from build123d import *

# Parameters (mm, degrees)
SKETCH3_R            = 2.75
BOSS_EXTRUDE1_DEPTH  = 3
SKETCH4_R            = 2.75
BOSS_EXTRUDE2_DEPTH  = 3
BOSS_EXTRUDE3_DEPTH  = 3
BOSS_EXTRUDE4_START  = -3
SKETCH6_R            = 2.75
BOSS_EXTRUDE4_DEPTH  = 3
CUT_EXTRUDE1_START   = -0.4
CUT_EXTRUDE1_DEPTH   = 0.4
CUT_EXTRUDE2_DEPTH   = 0.4
BOSS_EXTRUDE5_DEPTH  = 26
SKETCH11_W           = 1.5
SKETCH11_H           = 10.4
CUT_EXTRUDE4_DEPTH   = 9.5
SKETCH13_W           = 13.75
SKETCH13_H           = 0.5
BOSS_EXTRUDE6_DEPTH  = 1
BOSS_EXTRUDE7_DEPTH  = 1
BOSS_EXTRUDE8_DEPTH  = 3
CHAMFER1_SIZE        = 2
FILLET1_R            = 1
SKETCH16_W           = 26
SKETCH16_H           = 3
BOSS_EXTRUDE9_DEPTH  = 1
FILLET2_R            = 2
BOSS_EXTRUDE11_DEPTH = 2.4
BOSS_EXTRUDE12_DEPTH = 1
CUT_EXTRUDE5_DEPTH   = 0.5


with BuildPart() as part:
    # Sketch3 → Boss-Extrude1 (new body)
    with BuildSketch(Plane(origin=(10, 0, 0), x_dir=(0, 0, -1), z_dir=(1, 0, 0))):
        with BuildLine():
            Line((-37, 41.45), (-42, 41.45))
            Line((-42, 41.45), (-47, 41.45))
            Line((-47, 41.45), (-47, 34.45))
            ThreePointArc((-47, 34.45), (-46.121320344, 32.328679656), (-44, 31.45))
            Line((-44, 31.45), (-40, 31.45))
            ThreePointArc((-40, 31.45), (-37.878679656, 32.328679656), (-37, 34.45))
            Line((-37, 34.45), (-37, 41.45))
        make_face()
        with Locations((-42, 36.65)):
            Circle(SKETCH3_R, mode=Mode.SUBTRACT)
    extrude(amount=BOSS_EXTRUDE1_DEPTH)

    # Sketch6 → Boss-Extrude4 (add)
    with BuildSketch(Plane(origin=(13, 0, 0), x_dir=(0, 0, -1), z_dir=(1, 0, 0)).offset(BOSS_EXTRUDE4_START)):
        with BuildLine():
            Line((-36.6, 31.45), (-36.6, 41.45))
            Line((-36.6, 41.45), (-47, 41.45))
            Line((-47, 41.45), (-47, 34.45))
            ThreePointArc((-47, 34.45), (-46.121320344, 32.328679656), (-44, 31.45))
            Line((-44, 31.45), (-36.6, 31.45))
        make_face()
        with Locations(Location((-42, 36.65, 0), (0, 0, 180))):
            Circle(SKETCH6_R, mode=Mode.SUBTRACT)
    extrude(amount=BOSS_EXTRUDE4_DEPTH)

    # Sketch8 → Cut-Extrude2 (cut)
    with BuildSketch(Plane.ZY.offset(-10)):
        with BuildLine():
            Line((47, 41.45), (36.6, 41.45))
            Line((36.6, 41.45), (36.6, 31.45))
            Line((36.6, 31.45), (44, 31.45))
            ThreePointArc((44, 31.45), (46.121320344, 32.328679656), (47, 34.45))
            Line((47, 34.45), (47, 41.45))
        make_face()
    extrude(amount=-CUT_EXTRUDE2_DEPTH, mode=Mode.SUBTRACT)



with BuildPart() as body_2:
    # Sketch4 → Boss-Extrude2 (new body)
    with BuildSketch(Plane.ZY.offset(10)):
        with BuildLine():
            Line((47, 41.45), (37, 41.45))
            Line((37, 41.45), (37, 34.45))
            ThreePointArc((37, 34.45), (37.878679656, 32.328679656), (40, 31.45))
            Line((40, 31.45), (44, 31.45))
            ThreePointArc((44, 31.45), (46.121320344, 32.328679656), (47, 34.45))
            Line((47, 34.45), (47, 41.45))
        make_face()
        with Locations((42, 36.65)):
            Circle(SKETCH4_R, mode=Mode.SUBTRACT)
    extrude(amount=BOSS_EXTRUDE2_DEPTH)

    # Sketch5 → Boss-Extrude3 (add)
    with BuildSketch(Plane.ZY.offset(13)):
        with BuildLine():
            Line((37, 41.45), (36.6, 41.45))
            Line((36.6, 41.45), (36.6, 31.45))
            Line((36.6, 31.45), (40, 31.45))
            ThreePointArc((40, 31.45), (37.878679656, 32.328679656), (37, 34.45))
            Line((37, 34.45), (37, 41.45))
        make_face()
    extrude(amount=-BOSS_EXTRUDE3_DEPTH)

    # Sketch7 → Cut-Extrude1 (cut)
    with BuildSketch(Plane(origin=(-10, 0, 0), x_dir=(0, 0, -1), z_dir=(1, 0, 0)).offset(CUT_EXTRUDE1_START)):
        with BuildLine():
            Line((-36.6, 41.45), (-47, 41.45))
            Line((-47, 41.45), (-47, 34.45))
            ThreePointArc((-47, 34.45), (-46.121320344, 32.328679656), (-44, 31.45))
            Line((-44, 31.45), (-36.6, 31.45))
            Line((-36.6, 31.45), (-36.6, 41.45))
        make_face()
    extrude(amount=CUT_EXTRUDE1_DEPTH, mode=Mode.SUBTRACT)


with BuildPart() as part_1:
    add(part.part)

    add(body_2.part)  # Boss-Extrude5 merges body 2
    # Sketch9 → Boss-Extrude5 (add)
    with BuildSketch(Plane(origin=(13, 0, 0), x_dir=(0, 0, -1), z_dir=(1, 0, 0))):
        with BuildLine():
            ThreePointArc((-31.6, 41.45), (-35.135533906, 39.985533906), (-36.6, 36.45))
            Line((-36.6, 36.45), (-34.35, 36.45))
            ThreePointArc((-34.35, 36.45), (-31.6, 39.2), (-28.85, 36.45))
            Line((-28.85, 36.45), (-26.6, 36.45))
            ThreePointArc((-26.6, 36.45), (-28.064466094, 39.985533906), (-31.6, 41.45))
        make_face()
        with BuildLine():
            Line((-34.35, 36.45), (-36.6, 36.45))
            ThreePointArc((-36.6, 36.45), (-35.135533906, 32.914466094), (-31.6, 31.45))
            ThreePointArc((-31.6, 31.45), (-28.064466094, 32.914466094), (-26.6, 36.45))
            Line((-26.6, 36.45), (-28.85, 36.45))
            ThreePointArc((-28.85, 36.45), (-31.6, 33.7), (-34.35, 36.45))
        make_face()
        with BuildLine():
            Line((-36.6, 41.45), (-36.6, 36.45))
            ThreePointArc((-36.6, 36.45), (-35.135533906, 39.985533906), (-31.6, 41.45))
            Line((-31.6, 41.45), (-36.6, 41.45))
        make_face()
        with BuildLine():
            Line((-36.6, 36.45), (-36.6, 31.45))
            Line((-36.6, 31.45), (-34.34369351, 31.45))
            Line((-34.34369351, 31.45), (-31.6, 31.45))
            ThreePointArc((-31.6, 31.45), (-35.135533906, 32.914466094), (-36.6, 36.45))
        make_face()
    extrude(amount=-BOSS_EXTRUDE5_DEPTH)

    # Sketch11 → Cut-Extrude4 (cut, symmetric)
    with BuildSketch(Plane.XY.offset(26.6)):
        with Locations((0, 36.65)):
            Rectangle(SKETCH11_W, SKETCH11_H)
    extrude(amount=CUT_EXTRUDE4_DEPTH, both=True, mode=Mode.SUBTRACT)



with BuildPart() as body_2_2:
    # Sketch13 → Boss-Extrude6 (new body)
    with BuildSketch(Plane(origin=(0, 31.05, 0), x_dir=(-1, 0, 0), z_dir=(0, -1, 0))):
        Polygon((-0.75, -36.6), (-10.4, -36.6), (-13, -36.6), (-13, -41.6), (13, -41.6), (13, -36.6), align=None)
        with Locations((6.125, -36.35)):
            Rectangle(SKETCH13_W, SKETCH13_H)
        Polygon((-13, -36.6), (-10.4, -36.6), (-0.75, -36.6), (-0.75, -36.1), (-13, -36.1), align=None)
    extrude(amount=BOSS_EXTRUDE6_DEPTH)


with BuildPart() as part_2:
    add(part_1.part)

    add(body_2_2.part)  # Boss-Extrude7 merges body 2 2
    # Sketch14 → Boss-Extrude7 (add)
    with BuildSketch(Plane.XZ.offset(-31.45)):
        Polygon((10.4, 41.6), (13, 41.6), (13, 36.1), (-13, 36.1), (-13, 41.6), (-10.4, 41.6), (-10.4, 36.6), (10.4, 36.6), align=None)
    extrude(amount=BOSS_EXTRUDE7_DEPTH)

    # Sketch15 → Boss-Extrude8 (add)
    with BuildSketch(Plane(origin=(0, 41.45, 0), x_dir=(1, 0, 0), z_dir=(0, 1, 0))):
        Polygon((-10.4, -36.6), (10.4, -36.6), (13, -36.6), (13, -34.6), (0.75, -34.6), (0.75, -36.1), (-0.75, -36.1), (-0.75, -34.6), (-13, -34.6), (-13, -36.6), align=None)
    extrude(amount=BOSS_EXTRUDE8_DEPTH)

    # Chamfer1
    chamfer1_edges = [part_2.edges().sort_by_distance(p)[0] for p in [
        (-6.875, 41.45, 34.6),
        (6.875, 41.45, 34.6),
    ]]
    chamfer(chamfer1_edges, length=CHAMFER1_SIZE)

    # Fillet1
    fillet1_edges = [part_2.edges().sort_by_distance(p)[0] for p in [
        (-6.875, 44.45, 34.6),
        (6.875, 44.45, 34.6),
    ]]
    fillet(fillet1_edges, radius=FILLET1_R - 0.0001)  # a hair under: the kernel refuses the full size

    # Sketch16 → Boss-Extrude9 (add)
    with BuildSketch(Plane.XY.offset(36.6)):
        with Locations((0, 42.95)):
            Rectangle(SKETCH16_W, SKETCH16_H)
    extrude(amount=BOSS_EXTRUDE9_DEPTH)

    # Fillet2
    fillet2_edges = [part_2.edges().sort_by_distance(p)[0] for p in [
        (-11.7, 41.45, 47),
        (11.7, 41.45, 47),
    ]]
    fillet(fillet2_edges, radius=FILLET2_R)

    # Sketch17 → Boss-Extrude11 (add)
    with BuildSketch(Plane.XY.offset(41.6)):
        Polygon((10.4, 31.05), (-10.4, 31.05), (-10.4, 31.45), (-13, 31.45), (-13, 30.05), (13, 30.05), (13, 31.45), (10.4, 31.45), align=None)
    extrude(amount=BOSS_EXTRUDE11_DEPTH)

    # Sketch18 → Boss-Extrude12 (add)
    with BuildSketch(Plane.XY.offset(37.6)):
        Polygon((-13, 44.45), (-13, 41.45), (-10.4, 41.45), (10.4, 41.45), (13, 41.45), (13, 44.45), align=None)
    extrude(amount=BOSS_EXTRUDE12_DEPTH)

    # Sketch19 → Cut-Extrude5 (cut)
    with BuildSketch(Plane.XY.offset(38.6)):
        Polygon((13, 44.45), (-13, 44.45), (-13, 41.45), (-10.4, 41.45), (10.4, 41.45), (13, 41.45), align=None)
    extrude(amount=-CUT_EXTRUDE5_DEPTH, mode=Mode.SUBTRACT)


solid = part_2.part
Geometry: final body of the model. Coordinates: model frame, mm. A direction names the side the tool comes from. Round coordinates to 2 decimals unless told otherwise and drop trailing zeros. Loops run counter-clockwise (first coordinate to the right, second up) from the corner with the lowest first, then second, coordinate; pieces in that order, holes last.
Q1. Material intervals for L1, parallel to Z at x = -12.2, y = 36.65; L2, parallel to X at y = 37.5, z = 28.5; L3, parallel to X at y = 31.75, z = 44.25, sorted ascending.
Q2. Pin query (flat end, axial travel): P1, Ø0.8, axis at x = -5.5, z = 32, coming from the +Y side; P2, Ø1, axis at x = 4, z = 31.5, coming from the -Y side; P3, Ø3, axis at y = 38, z = 43, coming from the +X side; P4, Ø4, axis at x = 1.5, z = 32, coming from the +Y side. Return the tip coordinate at first contact, or that it passes through.
Q3. Section C-C on y = 38. Return loops of the section in (x, z).
Q4. Pull-direction query (X, two-part tool) for faces 1 (the flat face through (7, 41.45, 32)), 2 (the flat face through (13, 36, 37)), 3 (the flat face through (0, 41.45, 37)); classes: released by +X, released by -X, zero draft, split by the parting line, or undercut.
Q5. Section B-B on z = 42. Return loops of the section in (x, y).
Q6. Section D-D on z = 33.75. Return loops of the section in (x, y).
Q7. Access query for faces 4 (the flat face through (-7, 41.45, 32)), 5 (the flat face through (-12, 41.45, 42)), 6 (the flat face through (-10.4, 35, 39)), 7 (the flat face through (7, 31.45, 34)), 8 (the flat face through (-0.2, 30.6, 44)). Directions: +Z, -Z, +X, -X, +Y, -Y. A direction counts if a zero-diameter tool reaches every point of the face in a straight line with its end or side. Return the directions, or none.
Evaluation:
1. L1: z = 26.6 to 28.86, 34.34 to 39.25, 44.75 to 47
1. L2: x = -13 to -0.75, 0.75 to 13
1. L3: x = -13 to -10.4, 10.4 to 13
2. P1: stops at y = 41.45
2. P2: stops at y = 31.45
2. P3: stops at x = 13
2. P4: stops at y = 42.85
3. outline: (-13, 26.85) - (-0.75, 26.85) - (-0.75, 29.33) - (-13, 29.33) - close; (-13, 33.87) - (-0.75, 33.87) - (-0.75, 36.1) - (0.75, 36.1) - (0.75, 33.87) - (13, 33.87) - (13, 39.6) - (10.4, 39.6) - (10.4, 36.6) - (-10.4, 36.6) - (-10.4, 39.6) - (-13, 39.6) - close; (-13, 44.4) - (-10.4, 44.4) - (-10.4, 47) - (-13, 47) - close; (0.75, 26.85) - (13, 26.85) - (13, 29.33) - (0.75, 29.33) - close; (10.4, 44.4) - (13, 44.4) - (13, 47) - (10.4, 47) - close
4. face 1: zero draft
4. face 2: released by +X
4. face 3: undercut
5. outline: (-13, 30.05) - (13, 30.05) - (13, 33.9) - (10.4, 33.9) - (10.4, 31.05) - (-10.4, 31.05) - (-10.4, 33.9) - (-13, 33.9) - close; (-13, 39.4) - (-10.4, 39.4) - (-10.4, 41.45) - (-13, 41.45) - close; (10.4, 39.4) - (13, 39.4) - (13, 41.45) - (10.4, 41.45) - close
6. outline: (-13, 31.45) - (-0.75, 31.45) - (-0.75, 34.74) - (-13, 34.74) - close; (-13, 38.16) - (-0.75, 38.16) - (-0.75, 42.6) - (-13, 42.6) - close; (0.75, 31.45) - (13, 31.45) - (13, 34.74) - (0.75, 34.74) - close; (0.75, 38.16) - (13, 38.16) - (13, 42.6) - (0.75, 42.6) - close
7. face 4: -Z, +X, -X, +Y
7. face 5: +Z, +X, -X, +Y
7. face 6: +Z
7. face 7: -Z, +X, -X, -Y
7. face 8: +Z, +X, -X, -Y
